Geometry: final body of the model. Coordinates: model frame, mm. A direction names the side the tool comes from. Round coordinates to 2 decimals unless told otherwise and drop trailing zeros. Order: outer loops, then holes, each group sorted by start corner. A loop starts at its lowest first (then second) coordinate and runs counter-clockwise, first axis right, second up. Notation, with made-up numbers: M 80,-15.5 L 124,-15.5 A34 ccw 124,20.5 Z; hole C 86,3 d5. An arc over 180 degrees is marked long. Put each result on its own line as item: value. Start each with the question number.
1) Draft query along Z for faces 1 (the cylindrical face through (2.5, 30.8, 13.1)), 2 (the cylindrical face through (2.465, -36.347, 15.136)), 3 (the flat face through (20, 26.5, 5)), 4 (the flat face through (2, -31, 30)). Return one class per face: pulls with the +Z half, pulls with the -Z half, needs draft (parallel to the pull), parting line crosses it, or undercut.
2) Material intervals for probe 1 along Y at (x, z) = (-15, -2); probe 2 along Y at (x, z) = (37.5, -1.4); probe 3 along Y at (x, z) = (2.9, 15), sorted ascending. Write a range as [from, to].
3) Section A-A, the plane x = -15. Return loops of the section in (y, z), then the cut area to 3 significant figures.
4) Access query for faces 5 (the flat face through (20, -26.5, 8)), 6 (the flat face through (5, 30.6, 12.7)), 7 (the flat face through (-2, 1, 0)), 8 (the cylindrical face through (37.292, -13.914, -2.465)), 9 (the flat face through (0, 29, 15)). Directions: +Z, -Z, +X, -X, +Y, -Y. A direction counts if a zero-diameter tool reaches every point of the face in a straight line with its end or side. Return the directions, or none.
5) First-contact query: P1, Ø3.5, axis at x = 6.5, y = -15.5, coming from the +Z side; P2, Ø5, axis at y = -35.5, z = 12, coming from the -X side; P3, Ø7, axis at x = -15, y = 30, coming from the -Z side; P4, Ø12.5, axis at y = -36, z = 14, coming from the +X side. Flat tips, straight axial feed; report the tip coordinate or a pass-through.
6) Section B-B, the plane z = 15. Return loops of the section in (x, y).
7) Section C-C, the plane z = 10.5. Return loops of the section in (x, y), then the cut area to 3 significant figures.
8) Section D-D, the plane y = 15.5. Return loops of the section in (x, z).
from build123d import *

# Parameters (mm, degrees)
SKETCH_R             = 11.1
SKETCH_R_2           = 3.1
SKETCH_R_3           = 1.6
PAD_DEPTH            = 5
PAD001_DEPTH         = 30
SKETCH002_R          = 3.1
POCKET_DEPTH         = 43.001
POCKET001_DEPTH      = 40.001
POCKET001_DEPTH_BACK = -40.001
FILLET_R             = 1
SKETCH004_R          = 0.5
POCKET002_DEPTH      = 5.001
POCKET002_DEPTH_BACK = -30.001


with BuildPart() as part:
    # Sketch → Pad (new body)
    with BuildSketch(Plane.XY):
        Polygon((-30, 40), (-30, -40), (5, -40), (5, -26.5), (43, -26.5), (43, 26.5), (5, 26.5), (5, 40), align=None)
        with Locations((22, 0)):
            Circle(SKETCH_R, mode=Mode.SUBTRACT)
        with Locations((-15, 30)):
            Circle(SKETCH_R_2, mode=Mode.SUBTRACT)
        with Locations((-15, -30)):
            Circle(SKETCH_R_2, mode=Mode.SUBTRACT)
        with Locations((6.5, -15.5)):
            Circle(SKETCH_R_3, mode=Mode.SUBTRACT)
        with Locations((37.5, -15.5)):
            Circle(SKETCH_R_3, mode=Mode.SUBTRACT)
        with Locations((37.5, 15.5)):
            Circle(SKETCH_R_3, mode=Mode.SUBTRACT)
        with Locations((6.5, 15.5)):
            Circle(SKETCH_R_3, mode=Mode.SUBTRACT)
    extrude(amount=-PAD_DEPTH)

    # Sketch001 → Pad001 (join)
    with BuildSketch(Plane.XY):
        Polygon((0, -40), (5, -40), (5, -26.5), (43, -26.5), (43, -21.5), (0, -21.5), align=None)
        Polygon((0, 21.5), (43, 21.5), (43, 26.5), (5, 26.5), (5, 40), (0, 40), align=None)
    extrude(amount=PAD001_DEPTH)

    # Sketch002 → Pocket (cut, through all)
    with BuildSketch(Plane.YZ):
        with Locations((-33.25, 15)):
            Circle(SKETCH002_R)
        with Locations((33.25, 15)):
            Circle(SKETCH002_R)
    extrude(amount=POCKET_DEPTH, mode=Mode.SUBTRACT)

    # Sketch003 → Pocket001 (cut, two sides)
    with BuildSketch(Plane.XZ) as pocket001_sk:
        Polygon((5, 30), (43, 30), (43, 0), align=None)
    extrude(amount=-POCKET001_DEPTH, mode=Mode.SUBTRACT)
    extrude(pocket001_sk.sketch, amount=-POCKET001_DEPTH_BACK, mode=Mode.SUBTRACT)

    # Fillet
    fillet_edges = [part.edges().sort_by_distance(p)[0] for p in [
        (5, -26.5, 12.5),
        (5, 26.5, 12.5),
        (43, 26.5, -2.5),
        (43, -26.5, -2.5),
        (0, -21.5, 15),
        (0, 21.5, 15),
        (5, -40, 12.5),
        (5, 40, 12.5),
        (-30, 40, -2.5),
        (-30, -40, -2.5),
    ]]
    fillet(fillet_edges, radius=FILLET_R)

    # Sketch004 (on Face2 of Fillet) → Pocket002 (cut, two sides)
    with BuildSketch(Plane.XY) as pocket002_sk:
        with Locations((-30, 0)):
            Circle(SKETCH004_R)
    extrude(amount=-POCKET002_DEPTH, mode=Mode.SUBTRACT)
    extrude(pocket002_sk.sketch, amount=-POCKET002_DEPTH_BACK, mode=Mode.SUBTRACT)


solid = part.part
Result sheet:
1. face 1: undercut
1. face 2: undercut
1. face 3: needs draft
1. face 4: pulls with the +Z half
2. probe 1: y = [-40, -33.1], [-26.9, 26.9], [33.1, 40]
2. probe 2: y = [-26.5, -17.1], [-13.9, 13.9], [17.1, 26.5]
2. probe 3: y = [-40, -36.35], [-30.15, -21.5], [21.5, 30.15], [36.35, 40]
3. outline: M -40,-5 L -33.1,-5 L -33.1,0 L -40,0 Z; M -26.9,-5 L 26.9,-5 L 26.9,0 L -26.9,0 Z; M 33.1,-5 L 40,-5 L 40,0 L 33.1,0 Z
3. area: 338 mm2
4. face 5: +Z, -Z, +X, -Y
4. face 6: +Z, -Z, +X, +Y
4. face 7: +Z, -X
4. face 8: +Z, -Z
4. face 9: +Z, -X, +Y, -Y
5. P1: stops at z = 0
5. P2: stops at x = 0
5. P3: stops at z = -5
5. P4: stops at x = 5
6. outline: M 0,-40 L 4,-40 A1 ccw 5,-39 L 5,-36.35 L 0,-36.35 Z; M 0,-30.15 L 5,-30.15 L 5,-27.5 A1 cw 6,-26.5 L 24,-26.5 L 24,-21.5 L 1,-21.5 A1 ccw 0,-22.5 Z; M 0,22.5 A1 ccw 1,21.5 L 24,21.5 L 24,26.5 L 6,26.5 A1 cw 5,27.5 L 5,30.15 L 0,30.15 Z; M 0,36.35 L 5,36.35 L 5,39 A1 ccw 4,40 L 0,40 Z
7. outline: M 0,-40 L 4,-40 A1 ccw 5,-39 L 5,-27.5 A1 cw 6,-26.5 L 29.7,-26.5 L 29.7,-21.5 L 1,-21.5 A1 ccw 0,-22.5 Z; M 0,22.5 A1 ccw 1,21.5 L 29.7,21.5 L 29.7,26.5 L 6,26.5 A1 cw 5,27.5 L 5,39 A1 ccw 4,40 L 0,40 Z
7. area: 432 mm2
8. outline: M -30,-5 L 4.9,-5 L 4.9,0 L -30,0 Z; M 8.1,-5 L 35.9,-5 L 35.9,0 L 8.1,0 Z; M 39.1,-5 L 43,-5 L 43,0 L 39.1,0 Z
